Read the model definition and answer for the solid it produces. Units are mm, in the model's axes. A direction names the side the tool comes from. Give positions to 0.01 mm unless a question says otherwise; leave off trailing zeros. Write each loop counter-clockwise with the first axis right and the second up, starting at its lowest first coordinate (ties: lowest second). Pieces come first, ordered by that corner, then holes. Notation, with made-up numbers: (73, 19) - (90, 19) arc R22 cw to (90, 42) - close; hole circle Ø6 at (-30, 65.5). An arc over 180 degrees is marked (long way). Answer as CSV lines item,"result".
```python
from build123d import *

# Parameters (mm, degrees)
SKETCH093_R            = 1.5
PAD070_DEPTH           = 100
CYLINDER003_R          = 6
CYLINDER003_DEPTH      = 80
CYLINDER003_ROLL_ANGLE = -90
CYLINDER004_R          = 18
CYLINDER004_DEPTH      = 52.25
CYLINDER004_ROLL_ANGLE = -90
CHAMFER005_SIZE        = 3
SKETCH060_W            = 30
SKETCH060_H            = 2
PAD043_DEPTH           = 100
ARRAY001_Y_COUNT       = 15
ARRAY001_Y_PITCH       = 7
SKETCH059_W            = 20.84431
SKETCH059_H            = 42
PAD042_DEPTH           = 10
SKETCH062_R            = 1.7
PAD045_DEPTH           = 40
PAD044_DEPTH           = 13
PAD068_DEPTH           = 6
SKETCH090_R            = 1.7
PAD067_DEPTH           = 100
SKETCH089_R            = 1.5
PAD066_DEPTH           = 3
PAD065_DEPTH           = 3
SKETCH092_R            = 1.5
SKETCH092_W            = 2.5
SKETCH092_H            = 5
PAD069_DEPTH           = 3


with BuildPart() as pad070:
    # Sketch093 → Pad070 (new body)
    with BuildSketch(Plane.XY):
        with Locations((0, 86)):
            Circle(SKETCH093_R)
        with Locations((0, 26)):
            Circle(SKETCH093_R)
    extrude(amount=PAD070_DEPTH)


with BuildPart() as obj1:
    # Cylinder003 → Cylinder003 (new body)
    with BuildSketch(Plane.XY):
        Circle(CYLINDER003_R)
    extrude(amount=CYLINDER003_DEPTH)


with BuildPart() as obj1_1:
    # Cylinder003 roll: moved
    add(obj1.part.rotate(Axis((0, 0, 0), (1, 0, 0)), CYLINDER003_ROLL_ANGLE))


with BuildPart() as obj1_2:
    # Cylinder003 placement: moved
    add(obj1_1.part)


with BuildPart() as motorcutout:
    # Cylinder004 → Cylinder004 (new body)
    with BuildSketch(Plane.XY):
        Circle(CYLINDER004_R)
    extrude(amount=CYLINDER004_DEPTH)


with BuildPart() as motorcutout_1:
    # Cylinder004 roll: moved
    add(motorcutout.part.rotate(Axis((0, 0, 0), (1, 0, 0)), CYLINDER004_ROLL_ANGLE))


with BuildPart() as motorcutout_2:
    # Cylinder004 placement: moved
    add(motorcutout_1.part.moved(Location((0, 30, 0))))

    # Chamfer005
    chamfer005_edges = [motorcutout_2.edges().sort_by_distance(p)[0] for p in [
        (-18, 30, 0),
        (-18, 82.25, 0),
    ]]
    chamfer(chamfer005_edges, length=CHAMFER005_SIZE)

    # Fusion004012: union obj1
    add(obj1_2.part)


with BuildPart() as fincutout:
    # Sketch060 → Pad043 (new body)
    with BuildSketch(Plane.XY):
        with Locations((0, 1)):
            Rectangle(SKETCH060_W, SKETCH060_H)
    extrude(amount=PAD043_DEPTH)

    # Array001 Y: FinCutout ×15


with BuildPart() as fincutout_1:
    add(fincutout.part)
    with Locations(*[(0, i * ARRAY001_Y_PITCH, 0) for i in range(1, ARRAY001_Y_COUNT)]):
        add(fincutout.part)


with BuildPart() as fincutout_2:
    # Array001 placement: moved
    add(fincutout_1.part.moved(Location((0, 2.5, 0))))


with BuildPart() as motormountfins:
    # Sketch059 → Pad042 (new body)
    with BuildSketch(Plane.XY.offset(20)):
        with Locations((0, 56)):
            Rectangle(SKETCH059_W, SKETCH059_H)
    extrude(amount=-PAD042_DEPTH)

    # Cut007012: cut FinCutout
    add(fincutout_2.part, mode=Mode.SUBTRACT)

    # Cut007013: cut MotorCutout
    add(motorcutout_2.part, mode=Mode.SUBTRACT)


with BuildPart() as motorscrewcutouts:
    # Sketch062 → Pad045 (new body)
    with BuildSketch(Plane.XZ):
        with Locations((-5.773925, 9.945441)):
            Circle(SKETCH062_R)
        with Locations((5.726042, 9.973086)):
            Circle(SKETCH062_R)
    extrude(amount=-PAD045_DEPTH)


with BuildPart() as motormountendcaps:
    # Sketch061 → Pad044 (new body)
    with BuildSketch(Plane.XY.offset(20)):
        with BuildLine():
            ThreePointArc((12.5, 83), (0, 89.708438), (-12.5, 83))
            Line((-12.5, 83), (12.5, 83))
        make_face()
        with BuildLine():
            Line((-12.5, 30), (12.5, 30))
            ThreePointArc((-12.5, 30), (0, 23.291562), (12.5, 30))
        make_face()
    extrude(amount=-PAD044_DEPTH)

    # Cut007015: cut MotorScrewCutouts
    add(motorscrewcutouts.part, mode=Mode.SUBTRACT)


with BuildPart() as pad068:
    # Sketch091 → Pad068 (new body)
    with BuildSketch(Plane.XY.offset(26)):
        with BuildLine():
            Line((-16.5, 15), (16.5, 15))
            Line((16.5, 15), (16.5, 82))
            ThreePointArc((16.5, 82), (0, 90.697345), (-16.5, 82))
            Line((-16.5, 82), (-16.5, 15))
        make_face()
    extrude(amount=-PAD068_DEPTH)


with BuildPart() as mountscrewcutouts:
    # Sketch090 → Pad067 (new body)
    with BuildSketch(Plane.XY):
        with Locations((28.75, 0)):
            Circle(SKETCH090_R)
        with Locations((18.75, 0)):
            Circle(SKETCH090_R)
    extrude(amount=PAD067_DEPTH)


with BuildPart() as baseplate:
    # Sketch089 → Pad066 (new body)
    with BuildSketch(Plane(origin=(0, 0, 23), x_dir=(-1, 0, 0), z_dir=(0, 0, 1))):
        Polygon((-31.5, -4), (-31.5, 4), (-16.5, 7.5), (0, 7.5), (0, -7.5), (-16.5, -7.5), align=None)
        with Locations((-5, 3)):
            Circle(SKETCH089_R, mode=Mode.SUBTRACT)
        with Locations((-5, -3)):
            Circle(SKETCH089_R, mode=Mode.SUBTRACT)
    extrude(amount=PAD066_DEPTH)


with BuildPart() as supportplate:
    # Sketch088 → Pad065 (new body)
    with BuildSketch(Plane(origin=(0, 0, 20), x_dir=(-1, 0, 0), z_dir=(0, 0, 1))):
        Polygon((-31.5, -4), (-31.5, 4), (-16.5, 7.5), (-16.5, -7.5), align=None)
    extrude(amount=PAD065_DEPTH)

    # Fusion004026: union BasePlate
    add(baseplate.part)

    # Cut007019005: cut MountScrewCutouts
    add(mountscrewcutouts.part, mode=Mode.SUBTRACT)


with BuildPart() as fusion004027:
    # Part__Mirroring002: instance of SupportPlate
    add(supportplate.part.mirror(Plane(origin=(0, 0, 0), x_dir=(0, -1, 0), z_dir=(1, 0, 0))))

    # Fusion004027: union SupportPlate
    add(supportplate.part)


with BuildPart() as obj2:
    # Sketch092 → Pad069 (new body)
    with BuildSketch(Plane.XY.offset(26)):
        with BuildLine():
            ThreePointArc((-15.611412, 76.887508), (-24.017848, 73.406119), (-27.5, 65))
            Line((-27.5, 2.5), (-27.5, 65))
            Line((27.5, 2.5), (-27.5, 2.5))
            Line((27.5, 65), (27.5, 2.5))
            ThreePointArc((27.5, 65), (24.018229, 73.405738), (15.612492, 76.887508))
            Line((-15.611412, 76.887508), (15.612492, 76.887508))
        make_face()
        with Locations((-22.5, 60)):
            Circle(SKETCH092_R, mode=Mode.SUBTRACT)
        with Locations((-22.5, 50)):
            Circle(SKETCH092_R, mode=Mode.SUBTRACT)
        with Locations((-22.5, 25)):
            Circle(SKETCH092_R, mode=Mode.SUBTRACT)
        with Locations((22.5, 60)):
            Circle(SKETCH092_R, mode=Mode.SUBTRACT)
        with Locations((22.5, 50)):
            Circle(SKETCH092_R, mode=Mode.SUBTRACT)
        with Locations((22.5, 25)):
            Circle(SKETCH092_R, mode=Mode.SUBTRACT)
        with Locations((-19.25, 67.5)):
            Rectangle(SKETCH092_W, SKETCH092_H, mode=Mode.SUBTRACT)
        with Locations((19.25, 67.5)):
            Rectangle(SKETCH092_W, SKETCH092_H, mode=Mode.SUBTRACT)
        with Locations((19.25, 37.5)):
            Rectangle(SKETCH092_W, SKETCH092_H, mode=Mode.SUBTRACT)
        with Locations((-19.25, 37.5)):
            Rectangle(SKETCH092_W, SKETCH092_H, mode=Mode.SUBTRACT)
    extrude(amount=-PAD069_DEPTH)

    # Fusion004028: union Pad068, Fusion004027
    add(pad068.part)
    add(fusion004027.part)

    # Fusion004029: union MotorMountFins, MotorMountEndCaps
    add(motormountfins.part)
    add(motormountendcaps.part)

    # Cut007019006: cut Pad070
    add(pad070.part, mode=Mode.SUBTRACT)


solid = obj2.part
```
(1) A cutting plane is placed at D-D (x = 0). Count the separate pieces of the cut face and the enclosed holes in it, and give its area (3 significant figures).
Worked out:
separate pieces,"3"
enclosed holes,"0"
area,"642 mm^2"
(2) A cutting plane is placed at A-A (y = 0). Write down the section's boundary in (x, z).
Worked out:
outline,"(-31.5, 20) - (-30.45, 20) - (-30.45, 26) - (-31.5, 26) - close; (-27.05, 20) - (-20.45, 20) - (-20.45, 26) - (-27.05, 26) - close; (-17.05, 20) - (-16.5, 20) - (-16.5, 23) - (16.5, 23) - (16.5, 20) - (17.05, 20) - (17.05, 26) - (-17.05, 26) - close; (20.45, 20) - (27.05, 20) - (27.05, 26) - (20.45, 26) - close; (30.45, 20) - (31.5, 20) - (31.5, 26) - (30.45, 26) - close"
(3) A cutting plane is placed at C-C (y = 57). Write down the section's boundary in (x, z), and give its area (3 significant figures).
Worked out:
outline,"(-27.5, 23) - (-16.5, 23) - (-16.5, 20) - (-10.42, 20) - (-10.42, 14.68) arc R18 cw to (10.42, 14.68) - (10.42, 20) - (16.5, 20) - (16.5, 23) - (27.5, 23) - (27.5, 26) - (-27.5, 26) - close"
area,"328 mm^2"
(4) Each of these flat-tipped pins is pushed along its axis until it touches: P1, Ø6, axis at x = 12.5, z = 12, coming from the +Y side; P2, Ø5.5, axis at y = 55.5, z = 18.5, coming from the -X side; P3, Ø3.5, axis at y = 67, z = 24.5, coming from the +X side; P4, Ø2.5, axis at x = -5, y = -3, coming from the -Z side. Where does it stop, or does it pass through?
Worked out:
P1,"stops at y = 86.32"
P2,"stops at x = -16.5"
P3,"stops at x = 27.5"
P4,"passes through"
(5) The mould has two halves that part along Z. Classify faces 1 (the flat face through (18, 67, 25)), 2 (the cylindrical face through (-4.152, 26.885, 10.456)), 3 (the flat face through (0, 84, 7)): +Z half, -Z half, draft (parallel to the pull), parting line (faces both ways), or undercut.
Worked out:
face 1,"draft"
face 2,"undercut"
face 3,"-Z half"
(6) For faces 4 (the flat face through (-16.5, 0, 21)), 5 (the flat face through (-0.1, 37.5, 18.5)), 6 (the flat face through (-20.5, 67, 25)), 7 (the cylindrical face through (0, 70, 18)), determine the directions among +Z, -Z, +X, -X, +Y, -Y from which every point of the face is accessible in a straight line to the end or side of a thin tool.
Worked out:
face 4,"-Z, -Y"
face 5,"-Z, +X, -X"
face 6,"+Z, -Z"
face 7,"-Z"
(7) A cutting plane is placed at B-B (x = -22.5). Write down the section's boundary in (y, z), and give its area (3 significant figures).
Worked out:
outline,"(-6.1, 20) - (6.1, 20) - (6.1, 23) - (23.5, 23) - (23.5, 26) - (-6.1, 26) - close; (26.5, 23) - (48.5, 23) - (48.5, 26) - (26.5, 26) - close; (51.5, 23) - (58.5, 23) - (58.5, 26) - (51.5, 26) - close; (61.5, 23) - (74.69, 23) - (74.69, 26) - (61.5, 26) - close"
area,"252 mm^2"
(8) Find the intervals of material crossed by L1, parallel to X at y = 0, z = 24.15; L2, parallel to X at y = 0, z = 22.45; L3, parallel to X at y = -3, z = 24.75, in increasing order.
Worked out:
L1,"x = -31.5 to -30.45, -27.05 to -20.45, -17.05 to 17.05, 20.45 to 27.05, 30.45 to 31.5"
L2,"x = -31.5 to -30.45, -27.05 to -20.45, -17.05 to -16.5, 16.5 to 17.05, 20.45 to 27.05, 30.45 to 31.5"
L3,"x = -31.5 to -6.5, -3.5 to 3.5, 6.5 to 31.5"
